Part model, mm, in its own coordinate system. A direction names the side the tool comes from. Round coordinates to 2 decimals unless told otherwise and drop trailing zeros. Order: outer loops, then holes, each group sorted by start corner. A loop starts at its lowest first (then second) coordinate and runs counter-clockwise, first axis right, second up. Notation, with made-up numbers: (-13, -15) - (12, -15) arc R23 ccw to (12, 21) - close; hole circle Ø6 at (65.25, 27). An arc over 180 degrees is marked (long way). Answer as a JSON object with one key per item and string values.
```python
from build123d import *

# Parameters (mm, degrees)
SKETCH1_R           = 15.24
SKETCH1_R_2         = 1.5875
BOSS_EXTRUDE1_DEPTH = 3.175
SKETCH1_3_R         = 1.5875
BOSS_EXTRUDE2_DEPTH = 6.35
CIRPATTERN1_COUNT   = 11


with BuildPart() as part:
    # Sketch1 → Boss-Extrude1 (new body)
    with BuildSketch(Plane.XY):
        Circle(SKETCH1_R)
        with Locations((0, 12.3825)):
            Circle(SKETCH1_R_2, mode=Mode.SUBTRACT)
        with BuildLine():
            Line((-1.1725, 0.975124992), (1.1725, 0.975124992))
            ThreePointArc((1.1725, 0.975124992), (0, -1.525), (-1.1725, 0.975124992))
        make_face(mode=Mode.SUBTRACT)
    extrude(amount=BOSS_EXTRUDE1_DEPTH)

    # Sketch1<3> → Boss-Extrude2 (add)
    with BuildSketch(Plane.XY):
        with Locations((0, 12.3825)):
            Circle(SKETCH1_3_R)
    boss_extrude2 = extrude(amount=BOSS_EXTRUDE2_DEPTH)

    # CirPattern1: Boss-Extrude2 ×11 about axis
    cirpattern1_axis = Axis((0, 0, 0), (0, 0, 1))
    for i in range(1, CIRPATTERN1_COUNT):
        add(boss_extrude2.rotate(cirpattern1_axis, i * 360 / CIRPATTERN1_COUNT))


solid = part.part
```
Item 1: Drop flat-ended pins along their axis: P1, Ø1.5, axis at y = -6.5, z = 5, coming from the +X side; P2, Ø1.8, axis at x = 0, y = 0, coming from the +Z side; P3, Ø1.5, axis at x = 1.5, y = 4, coming from the +Z side (3 decimals). Give the stop position or say it passes through.
Taken from the geometry:
{"P1": "x = 10.69", "P2": "through", "P3": "z = 3.175"}
Item 2: Cut at D-D (y = 5.5). Write the cut outline in (x, z) (3 decimals).
Taken from the geometry:
{"outline": "(-14.213, 0) - (14.213, 0) - (14.213, 3.175) - (12.811, 3.175) - (12.811, 6.35) - (9.716, 6.35) - (9.716, 3.175) - (-9.716, 3.175) - (-9.716, 6.35) - (-12.811, 6.35) - (-12.811, 3.175) - (-14.213, 3.175) - close"}
Item 3: Cut at C-C (y = -1). Write the cut outline in (x, z) (3 decimals), plus the area to 3 significant figures.
Taken from the geometry:
{"outline": "(-15.207, 0) - (-1.151, 0) - (-1.151, 3.175) - (-10.864, 3.175) - (-10.864, 6.35) - (-13.649, 6.35) - (-13.649, 3.175) - (-15.207, 3.175) - close; (1.151, 0) - (15.207, 0) - (15.207, 3.175) - (13.649, 3.175) - (13.649, 6.35) - (10.864, 6.35) - (10.864, 3.175) - (1.151, 3.175) - close", "area": "107 mm2"}
Item 4: Cut at A-A (x = 0). Write the cut outline in (y, z) (3 decimals).
Taken from the geometry:
{"outline": "(-15.24, 0) - (-1.525, 0) - (-1.525, 3.175) - (-15.24, 3.175) - close; (0.975, 0) - (15.24, 0) - (15.24, 3.175) - (13.97, 3.175) - (13.97, 6.35) - (10.795, 6.35) - (10.795, 3.175) - (0.975, 3.175) - close"}
Item 5: Tool access for faces 1 (the flat face through (0, 0.975, 2)), 2 (the cylindrical face through (-7.232, 8.923, 4.74)), 3 (the flat face through (-2, -3, 0)): list every direction of +Z, -Z, +X, -X, +Y, -Y with a clear straight run to the whole face (end or side of a thin tool).
Taken from the geometry:
{"face 1": "+Z, -Z", "face 2": "+Z", "face 3": "-Z, +X, -X, +Y, -Y"}
Item 6: Probe L1, parallel to Y at x = 0, z = 1.65 (3 decimals); L2, parallel to X at y = -8, z = 6; L3, parallel to Y at x = -3.5, z = 4.75. List the from-to ranges inside material, lowest first. Write a range as from..to.
Taken from the geometry:
{"L1": "-15.24..-1.525, 0.975..15.24", "L2": "-10.94..-7.77, 7.77..10.94", "L3": "-13.47..-10.29"}
Item 7: Two-plate mould, pull along X, no slides. Class faces 4 (the cylindrical face through (-3.3, -14.88, 1.57)), 5 (the flat face through (-12, -2, 6.35)), 6 (the cylindrical face through (-10.71, -7.28, 4.74)): pulls with the +X half, pulls with the -X half, needs draft (parallel to the pull), parting line crosses it, or undercut.
Taken from the geometry:
{"face 4": "parting line crosses it", "face 5": "needs draft", "face 6": "undercut"}
